Geometry check sheet. Reference: the model listing, model coordinates, mm. Coordinates: 2 decimals unless noted, no trailing zeros. Write each loop counter-clockwise with the first axis right and the second up, starting at its lowest first coordinate (ties: lowest second). Pieces come first, ordered by that corner, then holes. Notation, with made-up numbers: (15, 80.25) -> (38, 80.25) arc R28 cw to (38, 106.25) -> close; hole circle Ø10 at (70.25, -27.5). An arc over 180 degrees is marked (long way). Answer in a Markdown table with one row per item. Add a question column.
1. Cross-section at A-A on z = 16.5. Record the cut outline in (x, y), and give its area (3 significant figures).
2. Cross-section at C-C on z = 2. Record the cut outline in (x, y), and give its area (3 significant figures).
3. Cross-section at B-B on x = 8.5. Record the cut outline in (y, z).
4. Cross-section at D-D on y = -0.6. Give the number of separate pieces and of enclosed holes in the cut face, and give its area (3 significant figures).
5. Depth check by flat-ended pin: P1, Ø0.6, axis at x = 25.5, y = -0.5, coming from the -Z side. Enter the tip coordinate at first touch or a pass-through.
6. Scan lines: L1, parallel to X at y = -0.75, z = 23; L2, parallel to X at y = -0.1, z = -3; L3, parallel to X at y = -1.3, z = 14.5. Record each from-to range of solid material in increasing order. Write a range as from..to.
```python
from build123d import *

# Parameters (mm, degrees)
F0_R     = 1.6002
F0_R_2   = 2.375179
F1_DEPTH = 1.89738


with BuildPart() as f1:
    # F0 (on Front) → F1 (new body)
    with BuildSketch(Plane.XZ):
        with BuildLine():
            Line((30.804955, 27.38282), (-7.295045, 27.38282))
            Line((-7.295045, 27.38282), (-7.295045, 15.329635))
            ThreePointArc((-7.295045, 15.329635), (-6.365109, 13.084571), (-4.120045, 12.154635))
            Line((-4.120045, 12.154635), (0.667936, 12.154635))
            ThreePointArc((0.667936, 12.154635), (2.833681, 11.30131), (3.835278, 9.200021))
            Line((3.835278, 9.200021), (5.047635, -8.223763))
            Line((5.047635, -8.223763), (18.462275, -8.223763))
            Line((18.462275, -8.223763), (19.674632, 9.200021))
            ThreePointArc((19.674632, 9.200021), (20.676229, 11.30131), (22.841974, 12.154635))
            Line((22.841974, 12.154635), (27.629955, 12.154635))
            ThreePointArc((27.629955, 12.154635), (29.875019, 13.084571), (30.804955, 15.329635))
            Line((30.804955, 15.329635), (30.804955, 27.38282))
        make_face()
        with BuildLine():
            ThreePointArc((10.973398, -5.08104), (8.807653, -4.227715), (7.806056, -2.126426))
            Line((7.806056, -2.126426), (6.602346, 15.173074))
            ThreePointArc((6.602346, 15.173074), (7.448014, 17.559204), (9.769688, 18.568459))
            Line((9.769688, 18.568459), (13.755501, 18.568459))
            ThreePointArc((13.755501, 18.568459), (16.077176, 17.559204), (16.922843, 15.173074))
            Line((16.922843, 15.173074), (15.719134, -2.126426))
            ThreePointArc((15.719134, -2.126426), (14.717537, -4.227715), (12.551792, -5.08104))
            Line((12.551792, -5.08104), (10.973398, -5.08104))
        make_face(mode=Mode.SUBTRACT)
        with Locations((-4.120045, 15.329635)):
            Circle(F0_R, mode=Mode.SUBTRACT)
        with Locations((-4.120045, 22.467641)):
            Circle(F0_R_2, mode=Mode.SUBTRACT)
        with Locations((27.629955, 15.329635)):
            Circle(F0_R, mode=Mode.SUBTRACT)
        with Locations((27.629955, 22.467641)):
            Circle(F0_R_2, mode=Mode.SUBTRACT)
    extrude(amount=F1_DEPTH)


solid = f1.part
```
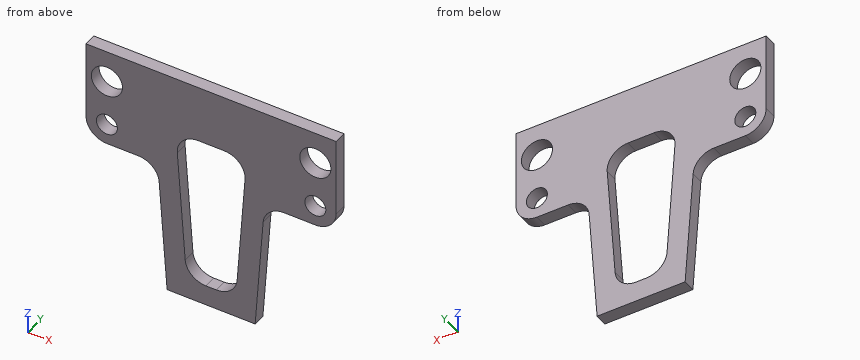
Results found:
| question | item | result |
|---|---|---|
| 1 | outline | (-7.3, -1.9) -> (-5.21, -1.9) -> (-5.21, 0) -> (-7.3, 0) -> close; (-3.03, -1.9) -> (6.79, -1.9) -> (6.79, 0) -> (-3.03, 0) -> close; (16.73, -1.9) -> (26.54, -1.9) -> (26.54, 0) -> (16.73, 0) -> close; (28.72, -1.9) -> (30.8, -1.9) -> (30.8, 0) -> (28.72, 0) -> close |
| 1 | area | 45.2 mm^2 |
| 2 | outline | (4.34, -1.9) -> (7.52, -1.9) -> (7.52, 0) -> (4.34, 0) -> close; (16.01, -1.9) -> (19.17, -1.9) -> (19.17, 0) -> (16.01, 0) -> close |
| 2 | area | 12.0 mm^2 |
| 3 | outline | (-1.9, -8.22) -> (0, -8.22) -> (0, -3.9) -> (-1.9, -3.9) -> close; (-1.9, 18.3) -> (0, 18.3) -> (0, 27.38) -> (-1.9, 27.38) -> close |
| 4 | separate pieces | 1 |
| 4 | enclosed holes | 5 |
| 4 | area | 623 mm^2 |
| 5 | P1 | stops at z = 12.15 |
| 6 | L1 | x = -7.3..-6.43, -1.81..25.32, 29.94..30.8 |
| 6 | L2 | x = 4.68..7.99, 15.53..18.83 |
| 6 | L3 | x = -7.18..-5.49, -2.75..6.65, 16.88..26.26, 29..30.69 |
